The listing builds one solid part. Answer for the finished solid, in the listing's coordinates (mm). A direction names the side the tool comes from. Give positions to 0.01 mm unless a question says otherwise; leave off trailing zeros. Return JSON: item names as keys, results as strings.
Autodesk Inventor part; units mm, degrees
ref_plane "YZ Plane" through (0, 0, 0) normal (1, 0, 0) x (0, 1, 0)
ref_plane "XZ Plane" through (0, 0, 0) normal (0, 1, 0) x (-1, 0, 0)
ref_plane "XY Plane" through (0, 0, 0) normal (0, 0, 1) x (1, 0, 0)
sketch "Sketch1" plane through (0, 0, 0) normal (0, 0, 1) x (1, 0, 0)
  line L0 (-2.205, 0) -> (2.205, 0)
  line L1 (0, -2.205) -> (0, 2.205)
  arc A0 (9, -10) -> (10, -9) centre (9, -9) ccw
  line L2 (-10, 9) -> (-10, 3)
  line L3 (-10, 3) -> (-8, 3)
  line L4 (-8, 3) -> (-8, 6)
  line L5 (-8, 6) -> (-7.0607, 6)
  line L6 (-7.0607, 6) -> (-4, 2.9393)
  line L7 (-4, 2.9393) -> (-4, 0.5196)
  line L8 (-4, 0.5196) -> (-3.7, 0)
  line L9 (-3.7, 0) -> (-4, -0.5196)
  line L10 (-4, -0.5196) -> (-4, -2.9393)
  line L11 (-4, -2.9393) -> (-7.0607, -6)
  line L12 (-7.0607, -6) -> (-8, -6)
  line L13 (-8, -6) -> (-8, -3)
  line L14 (-8, -3) -> (-10, -3)
  line L15 (-10, -3) -> (-10, -9)
  arc A1 (-10, -9) -> (-9, -10) centre (-9, -9) ccw
  line L16 (-9, -10) -> (-3, -10)
  line L17 (-3, -10) -> (-3, -8)
  line L18 (-3, -8) -> (-6, -8)
  line L19 (-6, -7.0607) -> (-2.9393, -4)
  line L20 (-2.9393, -4) -> (-0.5196, -4)
  line L21 (-0.5196, -4) -> (0, -3.7)
  line L22 (0, -3.7) -> (0.5196, -4)
  line L23 (0.5196, -4) -> (2.9393, -4)
  line L24 (2.9393, -4) -> (6, -7.0607)
  line L25 (6, -7.0607) -> (6, -8)
  line L26 (6, -8) -> (3, -8)
  line L27 (3, -8) -> (3, -10)
  line L28 (3, -10) -> (9, -10)
  line L29 (10, -9) -> (10, -3)
  line L30 (10, -3) -> (8, -3)
  line L31 (8, -3) -> (8, -6)
  line L32 (8, -6) -> (7.0607, -6)
  line L33 (7.0607, -6) -> (4, -2.9393)
  line L34 (4, -2.9393) -> (4, -0.5196)
  line L35 (4, -0.5196) -> (3.7, 0)
  line L36 (3.7, 0) -> (4, 0.5196)
  line L37 (4, 0.5196) -> (4, 2.9393)
  line L38 (4, 2.9393) -> (7.0607, 6)
  line L39 (7.0607, 6) -> (8, 6)
  line L40 (8, 6) -> (8, 3)
  line L41 (8, 3) -> (10, 3)
  line L42 (10, 3) -> (10, 9)
  arc A2 (10, 9) -> (9, 10) centre (9, 9) ccw
  line L43 (9, 10) -> (3, 10)
  line L44 (3, 10) -> (3, 8)
  line L45 (3, 8) -> (6, 8)
  line L46 (6, 8) -> (6, 7.0607)
  line L47 (6, 7.0607) -> (2.9393, 4)
  line L48 (2.9393, 4) -> (0.5196, 4)
  line L49 (0.5196, 4) -> (0, 3.7)
  line L50 (0, 3.7) -> (-0.5196, 4)
  line L51 (-0.5196, 4) -> (-2.9393, 4)
  line L52 (-2.9393, 4) -> (-6, 7.0607)
  line L53 (-6, 7.0607) -> (-6, 8)
  line L54 (-6, 8) -> (-3, 8)
  line L55 (-3, 8) -> (-3, 10)
  line L56 (-3, 10) -> (-9, 10)
  arc A3 (-9, 10) -> (-10, 9) centre (-9, 9) ccw
  circle A4 centre (0, 0) radius 2.1
  line L57 (-6, -8) -> (-6, -7.0607)
extrude "Extrusion1" add sketch "Sketch1" along normal mid plane 150
equation "\"d0\" = width"
equation "\"width\" = 150"
equation "\"panelChamfer\" = 75"
equation "\"suppourtPanelThickness\" = 2.38125"
properties part number "15 cm extrusion" material "Aluminum 6061"
Item 1: Find the intervals of material crossed by line 1 (X direction, y = 0, z = 27.5); line 2 (Y direction, x = -7.75, z = 38), in increasing order.
Geometry results:
{"line 1": "x = -3.7 to -2.1, 2.1 to 3.7", "line 2": "y = -10 to -6, 6 to 10"}
Item 2: Given pin 1 Ø2.5 at (y, z) = (-2, 30) entering from -X; pin 2 Ø0.6 at (x, z) = (9.5, -13.5) entering from -Y; pin 3 Ø2.5 at (y, z) = (1.5, -8.5) entering from +X; pin 4 Ø1 at (y, z) = (-1.5, 47) entering from -X, each flat-ended and moving along its own axis, determine where each tip first touches the part or whether it passes through.
Geometry results:
{"pin 1": "stops at x = -10", "pin 2": "stops at y = -9.98", "pin 3": "stops at x = 4", "pin 4": "stops at x = -4"}
Item 3: Which of the six approach directions +Z, -Z, +X, -X, +Y, -Y give full straight-line access (tool end or side, diameter ignored) to faces 1 (the flat face through (-0.1, 2.4, -75)), 2 (the flat face through (-8, -5, -1)), 3 (the flat face through (-4, 2, -1))?
Geometry results:
{"face 1": "-Z, +X, -X, +Y, -Y", "face 2": "+Z, -Z", "face 3": "+Z, -Z, -X"}
Item 4: Determine the mould class of faces 4 (the flat face through (-2, 4, -1)), 5 (the flat face through (-6, -10, -1)), 6 (the flat face through (10, -6, -1)) for opening direction X: +X half, -X half, draft (parallel to the pull), parting line (faces both ways), or undercut.
Geometry results:
{"face 4": "undercut", "face 5": "draft", "face 6": "+X half"}
